```python
from build123d import *

# Parameters (mm, degrees)
F0_W      = 450.85
F0_H      = 355.6
F1_DEPTH  = 79.375
F3_DEPTH  = 79.376
F4_R      = 12.7
F4_R_2    = 8.5328125
F5_DEPTH  = 38.1
F6_DEPTH  = 79.376
F7_R      = 6.35
F8_DEPTH  = 79.376
F9_R      = 6.35
F10_DEPTH = 79.376


with BuildPart() as f1:
    # F0 (on Top) → F1 (new body)
    with BuildSketch(Plane.XY):
        with Locations((-225.425, -177.8)):
            Rectangle(F0_W, F0_H)
    extrude(amount=-F1_DEPTH)

    # F2 (on face) → F3 (cut, through all)
    with BuildSketch(Plane.XY):
        with BuildLine():
            ThreePointArc((-40.4927648434, 0), (-18.3889970697, -26.3111717299), (0, -55.3404516789))
            Line((0, -55.3404516789), (0, 0))
            Line((0, 0), (-40.4927648434, 0))
        make_face()
        with BuildLine():
            Line((0, -355.6), (0, -300.2595483211))
            ThreePointArc((0, -300.2595483211), (-18.3889970697, -329.2888282701), (-40.4927648434, -355.6))
            Line((-40.4927648434, -355.6), (0, -355.6))
        make_face()
        with BuildLine():
            ThreePointArc((-410.3572351566, -355.6), (-225.425, -434.34), (-40.4927648434, -355.6))
            Line((-40.4927648434, -355.6), (-410.3572351566, -355.6))
        make_face()
        with BuildLine():
            ThreePointArc((-450.85, -55.3404516789), (-432.4610029303, -26.3111717299), (-410.3572351566, 0))
            Line((-410.3572351566, 0), (-450.85, 0))
            Line((-450.85, 0), (-450.85, -55.3404516789))
        make_face()
        with BuildLine():
            Line((-450.85, -355.6), (-410.3572351566, -355.6))
            ThreePointArc((-410.3572351566, -355.6), (-432.4610029303, -329.2888282701), (-450.85, -300.2595483211))
            Line((-450.85, -300.2595483211), (-450.85, -355.6))
        make_face()
    extrude(amount=-F3_DEPTH, mode=Mode.SUBTRACT)

    # F4 (on face) → F5 (cut)
    with BuildSketch(Plane.XY):
        with Locations((-385.445, -337.82)):
            Circle(F4_R)
        with Locations((-385.445, -337.82)):
            Circle(F4_R_2, mode=Mode.SUBTRACT)
        with Locations((-65.405, -17.78)):
            Circle(F4_R)
        with Locations((-65.405, -17.78)):
            Circle(F4_R_2, mode=Mode.SUBTRACT)
        with Locations((-65.405, -337.82)):
            Circle(F4_R)
        with Locations((-65.405, -337.82)):
            Circle(F4_R_2, mode=Mode.SUBTRACT)
        with Locations((-385.445, -17.78)):
            Circle(F4_R)
        with Locations((-385.445, -17.78)):
            Circle(F4_R_2, mode=Mode.SUBTRACT)
    extrude(amount=-F5_DEPTH, mode=Mode.SUBTRACT)

    # F4 (on face) → F6 (cut, through all)
    with BuildSketch(Plane.XY):
        with Locations((-385.445, -337.82)):
            Circle(F4_R_2)
        with Locations((-65.405, -337.82)):
            Circle(F4_R_2)
        with Locations((-65.405, -17.78)):
            Circle(F4_R_2)
        with Locations((-385.445, -17.78)):
            Circle(F4_R_2)
    extrude(amount=-F6_DEPTH, mode=Mode.SUBTRACT)

    # F7 (on face) → F8 (cut, through all)
    with BuildSketch(Plane.XY):
        with Locations((-377.825, -76.2)):
            Circle(F7_R)
        with Locations((-428.625, -76.2)):
            Circle(F7_R)
        with Locations((-327.025, -25.4)):
            Circle(F7_R)
        with Locations((-276.225, -25.4)):
            Circle(F7_R)
        with Locations((-225.425, -25.4)):
            Circle(F7_R)
        with Locations((-174.625, -25.4)):
            Circle(F7_R)
        with Locations((-123.825, -25.4)):
            Circle(F7_R)
        with Locations((-73.025, -76.2)):
            Circle(F7_R)
        with Locations((-123.825, -127)):
            Circle(F7_R)
        with Locations((-73.025, -127)):
            Circle(F7_R)
        with Locations((-22.225, -127)):
            Circle(F7_R)
        with Locations((-22.225, -76.2)):
            Circle(F7_R)
        with Locations((-123.825, -76.2)):
            Circle(F7_R)
        with Locations((-174.625, -76.2)):
            Circle(F7_R)
        with Locations((-225.425, -76.2)):
            Circle(F7_R)
        with Locations((-276.225, -76.2)):
            Circle(F7_R)
        with Locations((-327.025, -76.2)):
            Circle(F7_R)
        with Locations((-428.625, -127)):
            Circle(F7_R)
        with Locations((-327.025, -127)):
            Circle(F7_R)
        with Locations((-276.225, -127)):
            Circle(F7_R)
        with Locations((-225.425, -127)):
            Circle(F7_R)
        with Locations((-174.625, -127)):
            Circle(F7_R)
        with Locations((-225.425, -177.8)):
            Circle(F7_R)
        with Locations((-276.225, -177.8)):
            Circle(F7_R)
        with Locations((-327.025, -177.8)):
            Circle(F7_R)
        with Locations((-377.825, -177.8)):
            Circle(F7_R)
        with Locations((-428.625, -177.8)):
            Circle(F7_R)
        with Locations((-174.625, -177.8)):
            Circle(F7_R)
        with Locations((-73.025, -177.8)):
            Circle(F7_R)
        with Locations((-123.825, -177.8)):
            Circle(F7_R)
        with Locations((-22.225, -177.8)):
            Circle(F7_R)
        with Locations((-22.225, -228.6)):
            Circle(F7_R)
        with Locations((-123.825, -228.6)):
            Circle(F7_R)
        with Locations((-174.625, -228.6)):
            Circle(F7_R)
        with Locations((-73.025, -228.6)):
            Circle(F7_R)
        with Locations((-225.425, -228.6)):
            Circle(F7_R)
        with Locations((-276.225, -228.6)):
            Circle(F7_R)
        with Locations((-327.025, -228.6)):
            Circle(F7_R)
        with Locations((-377.825, -127)):
            Circle(F7_R)
        with Locations((-377.825, -228.6)):
            Circle(F7_R)
        with Locations((-428.625, -228.6)):
            Circle(F7_R)
        with Locations((-327.025, -279.4)):
            Circle(F7_R)
        with Locations((-377.825, -279.4)):
            Circle(F7_R)
        with Locations((-428.625, -279.4)):
            Circle(F7_R)
        with Locations((-276.225, -279.4)):
            Circle(F7_R)
        with Locations((-225.425, -279.4)):
            Circle(F7_R)
        with Locations((-22.225, -279.4)):
            Circle(F7_R)
        with Locations((-123.825, -330.2)):
            Circle(F7_R)
        with Locations((-174.625, -330.2)):
            Circle(F7_R)
        with Locations((-225.425, -330.2)):
            Circle(F7_R)
        with Locations((-174.625, -279.4)):
            Circle(F7_R)
        with Locations((-123.825, -279.4)):
            Circle(F7_R)
        with Locations((-73.025, -279.4)):
            Circle(F7_R)
        with Locations((-276.225, -330.2)):
            Circle(F7_R)
        with Locations((-327.025, -330.2)):
            Circle(F7_R)
    extrude(amount=-F8_DEPTH, mode=Mode.SUBTRACT)

    # F9 (on face) → F10 (cut, through all)
    with BuildSketch(Plane.XY):
        with Locations((-403.225, -304.8)):
            Circle(F9_R)
        with Locations((-352.425, -304.8)):
            Circle(F9_R)
        with Locations((-352.425, -50.8)):
            Circle(F9_R)
        with Locations((-403.225, -50.8)):
            Circle(F9_R)
        with Locations((-98.425, -50.8)):
            Circle(F9_R)
        with Locations((-47.625, -50.8)):
            Circle(F9_R)
        with Locations((-98.425, -304.8)):
            Circle(F9_R)
        with Locations((-47.625, -304.8)):
            Circle(F9_R)
    extrude(amount=-F10_DEPTH, mode=Mode.SUBTRACT)


solid = f1.part
```
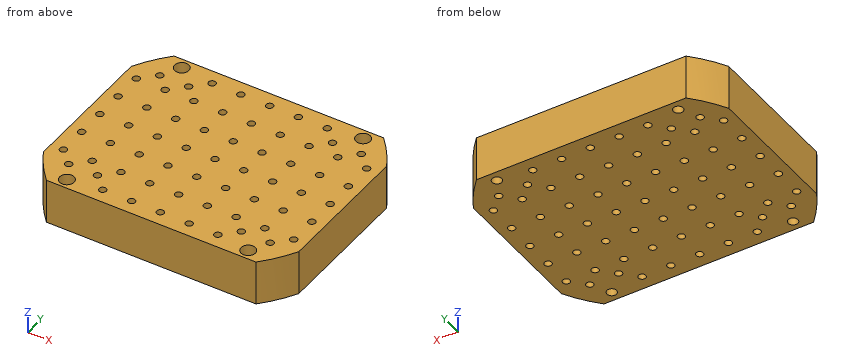
The listing builds one solid part. Answer for the finished solid, in the listing's coordinates (mm). Coordinates: 2 decimals unless noted, no trailing zeros. Write each loop counter-clockwise with the first axis right and the second up, starting at its lowest first coordinate (ties: lowest second). Pieces come first, ordered by that corner, then holes. Notation, with made-up numbers: (20, -6) -> (57, -6) arc R15 cw to (57, 20) -> close; hole circle Ø2 at (4.5, 38.25). An arc over 180 degrees is marked (long way). Write each question's results on one line, items separated by ' | '. Start each with the question number.
1) A cutting plane is placed at D-D (y = -38). Determine the outline of the cut face in (x, z) (3 decimals), then the cut area to 3 significant figures.
2) A cutting plane is placed at A-A (z = -16). Count the separate pieces of the cut face and the enclosed holes in it, then the cut area to 3 significant figures.
3) Straight lines are drawn through the part: probe 1 along Y at (x, z) = (-18.5, -25); probe 2 along Y at (x, z) = (-63, -68); probe 3 along Y at (x, z) = (-38, -58.5). For each, find the intervals that lie inside material, in ascending order.
4) Flat-ended cylindrical pins translate along their axes: pin 1 Ø11.5 at (x, y) = (-22.225, -177.8) entering from +Z; pin 2 Ø6 at (y, z) = (-42.5, -10) entering from +X; pin 3 Ø7.5 at (x, y) = (-70.5, -21) entering from +Z. Find the tip coordinate at first contact, or state that the pin passes through.
Values follow:
1) outline: (-440.527, -79.375) -> (-10.323, -79.375) -> (-10.323, 0) -> (-440.527, 0) -> close | area: 34,100 mm²
2) separate pieces: 1 | enclosed holes: 67 | area: 146,000 mm²
3) probe 1: -329.44 to -284.54, -274.26 to -233.74, -223.46 to -182.94, -172.66 to -132.14, -121.86 to -81.34, -71.06 to -26.16 | probe 2: -355.6 to -346.01, -329.63 to -25.97, -9.59 to 0 | probe 3: -352.97 to -2.63
4) pin 1: through | pin 2: x = -5.63 | pin 3: z = -38.1
